Autodesk Inventor part; units mm, degrees
ref_plane "YZ Plane" through (0, 0, 0) normal (1, 0, 0) x (0, 1, 0)
ref_plane "XZ Plane" through (0, 0, 0) normal (0, 1, 0) x (-1, 0, 0)
ref_plane "XY Plane" through (0, 0, 0) normal (0, 0, 1) x (1, 0, 0)
sketch "Sketch1" plane through (0, 0, 0) normal (0, 0, 1) x (1, 0, 0)
  line L0 (-15.2972, 20.3009) -> (-2.5972, 20.3009)
  line L1 (-2.5972, 20.3009) -> (-2.5972, -5.0991)
  line L2 (-1.0722, -17.7991) -> (-15.2972, -17.7991)
  line L3 (-15.2972, -17.7991) -> (-15.2972, 20.3009)
  line L4 (-2.5972, -5.0991) -> (21.4362, -5.0991)
  line L5 (21.4362, -5.0991) -> (21.4362, -17.7991)
  line L6 (21.4362, -17.7991) -> (-1.0722, -17.7991)
  point P0 (0, 0)
  dimension "d0" = 38.1
  dimension "d1" = 12.7
  dimension "d2" = 25.4
extrude "Extrusion1" add sketch "Sketch1" along normal blind 38.1
fillet "Fillet3" radius 6.35 3 edges at (-2.5972, 20.3009, 19.05) (-2.5972, -5.0991, 19.05) (21.4362, -5.0991, 19.05)
properties part number "FilletAngle"
Could you check a few things on this model? Use its own coordinates, in mm. A direction names the side the tool comes from. Round coordinates to 2 decimals unless told otherwise and drop trailing zeros. Order: outer loops, then holes, each group sorted by start corner. A loop starts at its lowest first (then second) coordinate and runs counter-clockwise, first axis right, second up.
Q1. Imagine slicing it at C-C, the plane x = 11. List the corners of the cut face in (y, z) for me, then the cut area to 3 significant figures.
Geometry says:
outline: (-17.8, 0) - (-5.1, 0) - (-5.1, 38.1) - (-17.8, 38.1) - close
area: 484 mm2
Q2. Which directions (+Z, -Z, +X, -X, +Y, -Y) give clear straight access to the entire face, cutting with the end or side of a thin tool? Please do faces 1 (the face through (21.436, -15, 19)), 2 (the face through (-2.597, 8, 19)).
Geometry says:
face 1: +Z, -Z, +X, +Y, -Y
face 2: +Z, -Z, +X, +Y
Q3. I'm going to push flat-ended pins straight in: P1, Ø3.5, axis at x = 10, z = 12, coming from the +Y side; P2, Ø4, axis at y = 4.5, z = 26, coming from the +X side; P3, Ø1.5, axis at x = -6, z = 21, coming from the +Y side. Where does each tip first touch, or does it pass through?
Geometry says:
P1: stops at y = -5.1
P2: stops at x = -2.6
P3: stops at y = 19.91
Q4. Please list where these lines run through material, in increasing order: probe 1 along X at (y, z) = (13, 10.5); probe 2 along Y at (x, z) = (9.5, 2.5); probe 3 along X at (y, z) = (19, 25).
Geometry says:
probe 1: x = -15.3 to -2.6
probe 2: y = -17.8 to -5.1
probe 3: x = -15.3 to -5.1
Q5. Imagine slicing it at B-B, the plane y = 7.5. List the corners of the cut face in (x, z) for me.
Geometry says:
outline: (-15.3, 0) - (-2.6, 0) - (-2.6, 38.1) - (-15.3, 38.1) - close
Q6. Imagine slicing it at A-A, the plane z = 27.5. List the corners of the cut face in (x, y) for me, then the cut area to 3 significant figures.
Geometry says:
outline: (-15.3, -17.8) - (21.44, -17.8) - (21.44, -11.45) arc R6.35 ccw to (15.09, -5.1) - (3.75, -5.1) arc R6.35 cw to (-2.6, 1.25) - (-2.6, 13.95) arc R6.35 ccw to (-8.95, 20.3) - (-15.3, 20.3) - close
area: 780 mm2
